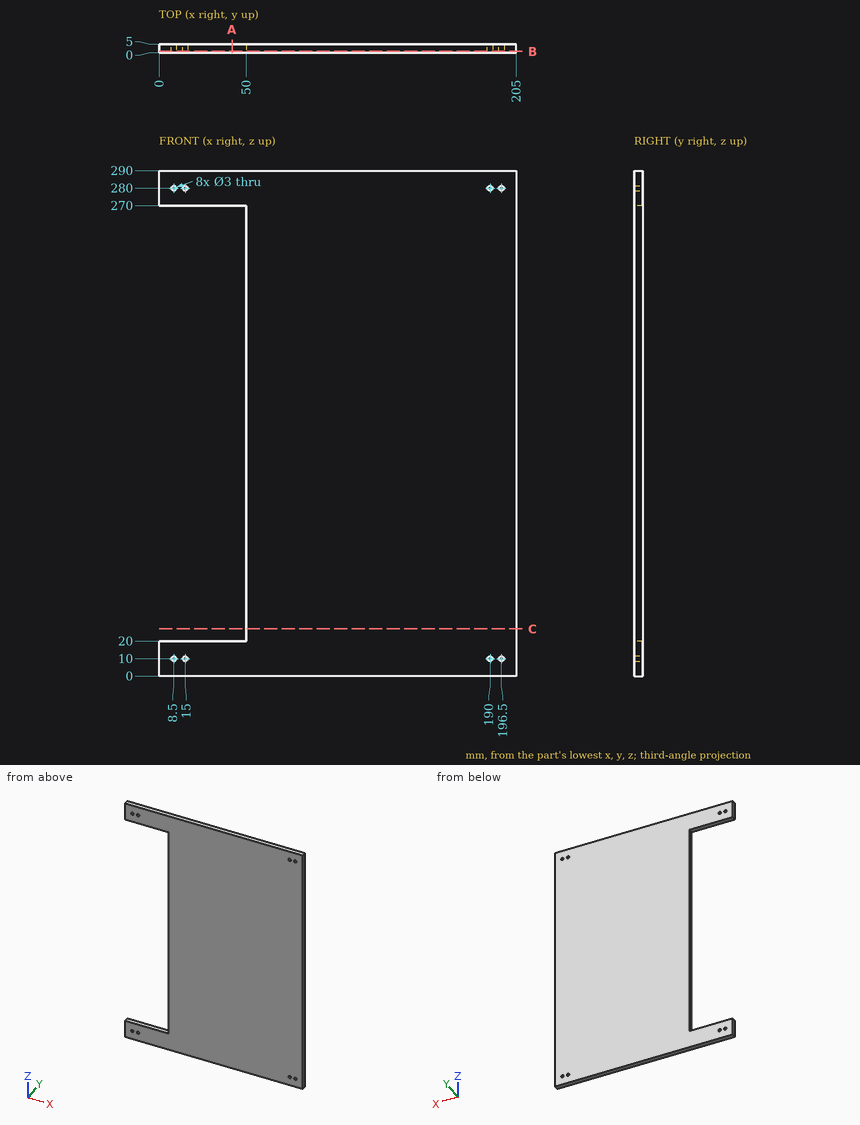
Input: dimensioned drawing with shaded views. Units: mm. Origin: part minimum x, y, z. Give positions to 0.01 mm unless a question says otherwise; leave off trailing zeros. Write each loop counter-clockwise with the first axis right and the second up, starting at its lowest first coordinate (ties: lowest second). Pieces come first, ordered by that corner, then holes. Notation, with made-up numbers: M 37,54 L 43,54 A11 cw 43,58 Z; hole C -15.75,54.25 d11. An arc over 180 degrees is marked long. Return JSON: item names as keys, results as strings. Group by question number.
1) Cut plane A-A, the plane x = 42. Output: boundary loops of the cut face in (y, z).
2) Material intervals for line 1 along X through (y, z) = (3.25, 10); line 2 along Z through (x, y) = (8.5, 1.45); line 3 along X through (y, z) = (2.9, 218), sorted ascending. Write a range as [from, to].
3) Cut plane C-C, the plane z = 27. Output: boundary loops of the cut face in (x, y), plus the area to 3 significant figures.
4) Cut plane B-B, the plane y = 0.8. Give the number of separate pieces and of enclosed holes in the cut face, plus the area to 3 significant figures.
5) Pin query (flat end, axial travel): P1, Ø2.5, axis at x = 196.5, z = 10, coming from the -Y side; P2, Ø2, axis at y = 1, z = 161.5, coming from the -X side. Return the tip coordinate at first contact, or that it passes through.
Recorded:
{
 "1": {"outline": "M 0,0 L 5,0 L 5,20 L 0,20 Z; M 0,270 L 5,270 L 5,290 L 0,290 Z"},
 "2": {"line 1": "x = [0, 7], [10, 13.5], [16.5, 188.5], [191.5, 195], [198, 205]", "line 2": "z = [0, 8.5], [11.5, 20], [270, 278.5], [281.5, 290]", "line 3": "x = [50, 205]"},
 "3": {"outline": "M 50,0 L 205,0 L 205,5 L 50,5 Z", "area": "775 mm²"},
 "4": {"separate pieces": "1", "enclosed holes": "8", "area": "46,900 mm²"},
 "5": {"P1": "passes through", "P2": "stops at x = 50"}
}
